Can you work these out from the model? Positions are in its coordinate system, mm. Face numbers are marked on the shaded views. A direction names the side the tool comes from. Round coordinates to 2 decimals unless told otherwise and drop trailing zeros. Write each loop counter-clockwise with the first axis right and the second up, starting at its lowest first coordinate (ties: lowest second). Pieces come first, ordered by that corner, then holes. Notation, with made-up numbers: (-31, -29) - (-14, -29) arc R10 cw to (-14, -22) - close; hole circle Ø8 at (74.5, 60.5). An arc over 180 degrees is marked (long way). One line per item, written item: value. Start each with the question number.
(1) If I drill on L1, parallel to X at y = 33, z = 250.5; L2, parallel to Y at x = -297, z = -210, over which ranges is the centre line in solid material (lowest first)? Write a range as from..to.
(2) I want a section at B-B on z = 210. List the corners of the cut face in (x, y) for me, plus the area to 3 significant figures.
(3) I want a section at C-C on x = 38. List the corners of the cut face in (y, z) for me, plus the area to 3 significant figures.
(4) I want a section at A-A on x = -70. List the corners of the cut face in (y, z) for me.
(5) I want a section at D-D on y = 209. List the corners of the cut face in (x, z) for me.
(6) On a 3-axis mill with a long thin cutter (end or side, diameter ignored), from which of +Z, -Z, +X, -X, +Y, -Y can I reach the whole of each face in a straight line? I mean the marked faces 4 and 5. Say none if no direction works.
(7) Thinking about a two-plate mould opening in Z: for the marked faces 1, 2 and 3, which applies, +Z half, -Z half, draft (parallel to the pull), parting line (faces both ways), or undercut?
Autodesk Inventor part; units mm, degrees
ref_plane "YZ Plane" through (0, 0, 0) normal (1, 0, 0) x (0, 1, 0)
ref_plane "XZ Plane" through (0, 0, 0) normal (0, 1, 0) x (-1, 0, 0)
ref_plane "XY Plane" through (0, 0, 0) normal (0, 0, 1) x (1, 0, 0)
sketch "Sketch1" plane through (0, 0, 0) normal (0, 1, 0) x (-1, 0, 0)
  line L0 (-280, 300) -> (280, 300)
  line L1 (300, 280) -> (300, -280)
  line L2 (280, -300) -> (-280, -300)
  line L3 (-300, -280) -> (-300, 280)
  line L4 (-300, 300) -> (300, -300) construction
  line L5 (300, 300) -> (-300, -300) construction
  arc A0 (300, 280) -> (280, 300) centre (280, 280) ccw
  arc A1 (280, -300) -> (300, -280) centre (280, -280) ccw
  arc A2 (-300, -280) -> (-280, -300) centre (-280, -280) ccw
  arc A3 (-280, 300) -> (-300, 280) centre (-280, 280) ccw
  line L6 (280, 294) -> (-280, 294)
  arc A4 (-280, 294) -> (-294, 280) centre (-280, 280) ccw
  line L7 (-294, 280) -> (-294, -280)
  arc A5 (-294, -280) -> (-280, -294) centre (-280, -280) ccw
  line L8 (-280, -294) -> (280, -294)
  arc A6 (280, -294) -> (294, -280) centre (280, -280) ccw
  line L9 (294, -280) -> (294, 280)
  arc A7 (294, 280) -> (280, 294) centre (280, 280) ccw
  point P0 (0, 0)
  dimension "d0" = 600
  dimension "d1" = 600
  dimension "d2" = 20
  dimension "d3" = 6
extrude "Extrusion1" add sketch "Sketch1" along normal blind 300
sketch "Sketch2" plane through (300, 0, 280) normal (1, 0, 0) x (0, 0, -1)
  line L0 (0, 0) -> (0, 300)
  line L1 (0, 150) -> (560, 150) construction
  line L2 (560, 0) -> (560, 300)
  point P0 (280, 0)
  point P1 (70, 150)
  point P2 (210, 150)
  point P3 (350, 150)
  point P4 (490, 150)
  dimension "d6" = 70
  dimension "d7" = 140
  dimension "d8" = 140
  dimension "d9" = 140
hole "Hole1" at (300, 150, 210) at (300, 150, 70) at (300, 150, -70) at (300, 150, -210) direction (-1, 0, 0) diameter 40 end through all
sketch "Sketch3" plane through (-280, 0, 300) normal (0, 0, 1) x (1, 0, 0)
  line L0 (0, 0) -> (0, 300)
  line L1 (0, 150) -> (560, 150) construction
  line L2 (560, 0) -> (560, 300)
  point P0 (280, 0)
  point P1 (70, 150)
  point P2 (210, 150)
  point P3 (350, 150)
  point P4 (490, 150)
  dimension "d17" = 70
  dimension "d18" = 140
  dimension "d19" = 140
  dimension "d20" = 140
hole "Hole2" at (-210, 150, 300) at (-70, 150, 300) at (70, 150, 300) at (210, 150, 300) direction (0, 0, -1) diameter 40 end through all
properties part number "Stackbox-40mm"
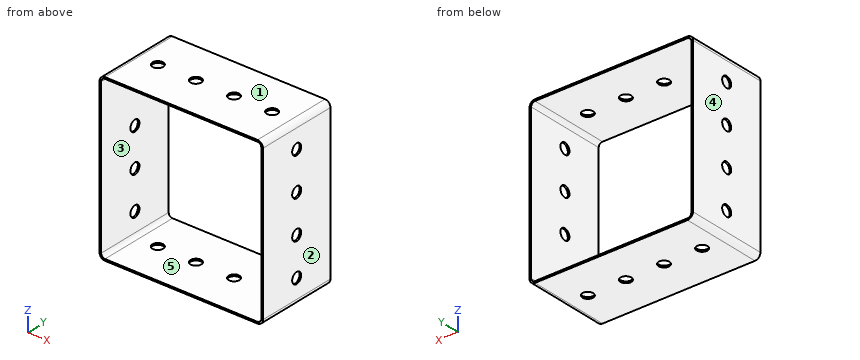
Established:
1. L1: -300..-294, 294..300
1. L2: 0..130, 170..300
2. outline: (-300, 0) - (-294, 0) - (-294, 130) - (-300, 130) - close; (-300, 170) - (-294, 170) - (-294, 300) - (-300, 300) - close; (294, 0) - (300, 0) - (300, 130) - (294, 130) - close; (294, 170) - (300, 170) - (300, 300) - (294, 300) - close
2. area: 3,120 mm2
3. outline: (0, -300) - (300, -300) - (300, -294) - (0, -294) - close; (0, 294) - (300, 294) - (300, 300) - (0, 300) - close
3. area: 3,600 mm2
4. outline: (0, -300) - (130, -300) - (130, -294) - (0, -294) - close; (0, 294) - (130, 294) - (130, 300) - (0, 300) - close; (170, -300) - (300, -300) - (300, -294) - (170, -294) - close; (170, 294) - (300, 294) - (300, 300) - (170, 300) - close
5. outline: (-300, -280) arc R20 ccw to (-280, -300) - (280, -300) arc R20 ccw to (300, -280) - (300, 280) arc R20 ccw to (280, 300) - (-280, 300) arc R20 ccw to (-300, 280) - close; hole (-294, -280) arc R14 ccw to (-280, -294) - (280, -294) arc R14 ccw to (294, -280) - (294, 280) arc R14 ccw to (280, 294) - (-280, 294) arc R14 ccw to (-294, 280) - close
6. face 4: +Z, -Z, -X, +Y, -Y
6. face 5: +Y, -Y
7. face 1: +Z half
7. face 2: draft
7. face 3: undercut
